Part model, mm, in its own coordinate system. A direction names the side the tool comes from. Coordinates: 2 decimals unless noted, no trailing zeros. Order: outer loops, then holes, each group sorted by start corner. A loop starts at its lowest first (then second) coordinate and runs counter-clockwise, first axis right, second up. Notation, with made-up numbers: (-28, 8) - (-19, 8) arc R18 ccw to (-19, 21) - close; hole circle Ø1 at (-23.5, 59.25). An arc over 180 degrees is marked (long way). Use a Markdown table: item, result. Add a question column.
1) Saw through at C-C on y = 4.5. List the corners of the cut face in (x, z), then the cut area to 3 significant figures.
2) Drop flat-ended pins along their axis: P1, Ø1.5, axis at x = 2.5, z = 3, coming from the +Y side; P2, Ø0.6, axis at x = -0.5, z = -21, coming from the +Y side. Give the stop position or say it passes through.
3) Saw through at A-A on y = 8.5. List the corners of the cut face in (x, z).
4) Wall check: L1, parallel to Z at x = -2.25, y = 11.5; L2, parallel to X at y = 4.5, z = -20.45; L3, parallel to Y at x = 0, z = 21.6. Give the ranges that are in metal, low to high. Write a range as [from, to].
5) Saw through at B-B on x = 0. List the corners of the cut face in (y, z).
6) Two-plate mould, pull along Y, no slides. Class faces 1 (the face through (-7.5, -1, 0)), 2 (the face through (-6.2, 3.6, 21)), 3 (the face through (-5.5, 13.9, 21)), 4 (the face through (6.386, 3.925, 20.986)): +Y half, -Y half, draft (parallel to the pull), parting line (faces both ways), or undercut.
7) Tool access for faces 5 (the face through (0, 0, 0)), 6 (the face through (0, 16, 21)), 7 (the face through (5.5, 13.9, 21)), 8 (the face through (0, 13, -21)): list every direction of +Z, -Z, +X, -X, +Y, -Y with a clear straight run to the whole face (end or side of a thin tool).
8) Saw through at D-D on y = 12. List the corners of the cut face in (x, z).
```python
from build123d import *

# Parameters (mm, degrees)
SALIENTE_EXTRUIR1_DEPTH    = 7.5
CORTAR_EXTRUIR1_DEPTH      = 29.217902119
CORTAR_EXTRUIR1_DEPTH_BACK = 29.217902119
CROQUIS2_R                 = 1.5
REDONDEO1_R                = 7


with BuildPart() as part:
    # Croquis1 → Saliente-Extruir1 (new, symmetric)
    with BuildSketch(Plane(origin=(0, 0, 0), x_dir=(0, 0, -1), z_dir=(1, 0, 0))):
        Polygon((-22, 13), (-22, -2), (22, -2), (22, 13), (20, 13), (20, 0), (-20, 0), (-20, 13), (-20, 16), (-22, 16), align=None)
    extrude(amount=SALIENTE_EXTRUIR1_DEPTH, both=True)

    # Croquis2 → Cortar-Extruir1 (cut, two sides: drawn at the far end of the back side and taken through both)
    with BuildSketch(Plane.XY.offset(-CORTAR_EXTRUIR1_DEPTH_BACK)):
        with Locations((0, 8.5)):
            Circle(CROQUIS2_R)
        with Locations((5, 4.5)):
            Circle(CROQUIS2_R)
        with Locations((-5, 4.5)):
            Circle(CROQUIS2_R)
    extrude(amount=CORTAR_EXTRUIR1_DEPTH + CORTAR_EXTRUIR1_DEPTH_BACK, mode=Mode.SUBTRACT)

    # Redondeo1
    redondeo1_edges = [part.edges().sort_by_distance(p)[0] for p in [
        (-7.5, 16, 21),
        (7.5, 16, 21),
    ]]
    fillet(redondeo1_edges, radius=REDONDEO1_R)


solid = part.part
```
Results are:
| question | item | result |
|---|---|---|
| 1 | outline | (-7.5, -22) - (-6.5, -22) - (-6.5, -20) - (-7.5, -20) - close; (-7.5, 20) - (-6.5, 20) - (-6.5, 22) - (-7.5, 22) - close; (-3.5, -22) - (3.5, -22) - (3.5, -20) - (-3.5, -20) - close; (-3.5, 20) - (3.5, 20) - (3.5, 22) - (-3.5, 22) - close; (6.5, -22) - (7.5, -22) - (7.5, -20) - (6.5, -20) - close; (6.5, 20) - (7.5, 20) - (7.5, 22) - (6.5, 22) - close |
| 1 | area | 36.0 mm2 |
| 2 | P1 | y = 0 |
| 2 | P2 | y = 13 |
| 3 | outline | (-7.5, -22) - (-1.5, -22) - (-1.5, -20) - (-7.5, -20) - close; (-7.5, 20) - (-1.5, 20) - (-1.5, 22) - (-7.5, 22) - close; (1.5, -22) - (7.5, -22) - (7.5, -20) - (1.5, -20) - close; (1.5, 20) - (7.5, 20) - (7.5, 22) - (1.5, 22) - close |
| 4 | L1 | [-22, -20], [20, 22] |
| 4 | L2 | [-7.5, -6.5], [-3.5, 3.5], [6.5, 7.5] |
| 4 | L3 | [-2, 7], [10, 16] |
| 5 | outline | (-2, -22) - (7, -22) - (7, -20) - (0, -20) - (0, 20) - (7, 20) - (7, 22) - (-2, 22) - close; (10, -22) - (13, -22) - (13, -20) - (10, -20) - close; (10, 20) - (16, 20) - (16, 22) - (10, 22) - close |
| 6 | face 1 | draft |
| 6 | face 2 | undercut |
| 6 | face 3 | +Y half |
| 6 | face 4 | undercut |
| 7 | face 5 | +X, -X, +Y |
| 7 | face 6 | +Z, -Z, +X, -X, +Y |
| 7 | face 7 | +Z, +X, +Y |
| 7 | face 8 | -Z, +X, -X, +Y |
| 8 | outline | (-7.5, -22) - (7.5, -22) - (7.5, -20) - (-7.5, -20) - close; (-6.82, 20) - (6.82, 20) - (6.82, 22) - (-6.82, 22) - close |
